Could you check a few things on this model? Use its own coordinates, in mm. Give positions to 0.01 mm unless a question says otherwise; leave off trailing zeros. Loops run counter-clockwise (first coordinate to the right, second up) from the corner with the lowest first, then second, coordinate; pieces in that order, holes last. Notation, with made-up numbers: M 36,57 L 45,57 A23 ccw 45,90 Z; hole C 64,85 d9. An arc over 180 degrees is marked long. Return JSON: item names as keys, results as strings. Group by question number.
1. If we section it at B-B (y = -64): Write out the boundary of the cut face in (x, z).
2. Please list where these lines run through material, in increasing order: line 1 (Z direction, x = 1.5, y = 6) (3 decimals); line 2 (Z direction, x = 1, y = 20); line 3 (Z direction, x = 1, y = -83.5).
3. If we section it at C-C (z = 23): Write out the boundary of the cut face in (x, y), plus the area to 3 significant figures.
4. If we section it at A-A (y = -19): Write out the boundary of the cut face in (x, z).
5. For pin 1 (1.3 mm diameter, centred on x = 3.5, z = 41, fed in from -Y); pin 2 (3 mm diameter, centred on x = 2, y = 4.5, fed in from -Z); pin 3 (0.7 mm diameter, centred on x = 2, z = 41, fed in from +Y), each with a flat end and sliding along its axis, tell me the tip position at first contact or that it passes through.
```python
from build123d import *

# Parameters (mm, degrees)
BOSS_EXTRUDE1_DEPTH = 6.35
CUT_EXTRUDE1_START  = -7.35
CUT_EXTRUDE1_DEPTH  = 8.35
LPATTERN1_COUNT     = 2
LPATTERN1_PITCH     = 19.05
CUT_EXTRUDE2_START  = -7.35
CUT_EXTRUDE2_DEPTH  = 8.35
CIRPATTERN2_COUNT   = 8
CIRPATTERN2_ANGLE   = 180
FILLET1_R           = 2.54


with BuildPart() as part:
    # Sketch1 → Boss-Extrude1 (new body)
    with BuildSketch(Plane(origin=(0, 0, 0), x_dir=(0, 0, -1), z_dir=(1, 0, 0))):
        with BuildLine():
            Line((-63.5, -98.425), (-63.5, 1.27))
            ThreePointArc((-63.5, 1.27), (-6.13650031, 61.522262538), (56.859225559, 7.185858903))
            Line((56.859225559, 7.185858903), (58.947868709, -14.009723349))
            ThreePointArc((58.947868709, -14.009723349), (54.036813814, -20.824301776), (46.661428403, -16.804273249))
            Line((46.661428403, -16.804273249), (35.802288852, 13.030967461))
            ThreePointArc((35.802288852, 13.030967461), (-6.615995569, 37.52117539), (-38.1, 0))
            Line((-38.1, 0), (-38.1, -98.425))
            ThreePointArc((-38.1, -98.425), (-50.8, -111.125), (-63.5, -98.425))
        make_face()
    extrude(amount=BOSS_EXTRUDE1_DEPTH)

    # Sketch4 → Cut-Extrude1 (cut)
    with BuildSketch(Plane(origin=(6.35, 0, 0), x_dir=(0, 0, -1), z_dir=(1, 0, 0)).offset(CUT_EXTRUDE1_START)):
        Polygon((44.489600492, -10.837225107), (47.473124563, -9.751311152), (45.301296653, -3.78426301), (42.317772582, -4.870176965), align=None)
    cut_extrude1 = extrude(amount=CUT_EXTRUDE1_DEPTH, mode=Mode.SUBTRACT)

    # LPattern1: Cut-Extrude1 ×2
    with Locations(*[Vector(0, 0.939692621, 0.342020143) * (i * LPATTERN1_PITCH) for i in range(1, LPATTERN1_COUNT)]):
        add(cut_extrude1, mode=Mode.SUBTRACT)

    # Sketch5 → Cut-Extrude2 (cut)
    with BuildSketch(Plane(origin=(6.35, 0, 0), x_dir=(0, 0, -1), z_dir=(1, 0, 0)).offset(CUT_EXTRUDE2_START)):
        Polygon((-38.1, 0), (-41.275, 0), (-41.275, 6.35), (-38.1, 6.35), (-35.06174314, 6.35), (-35.06174314, 0), align=None)
    cut_extrude2 = extrude(amount=CUT_EXTRUDE2_DEPTH, mode=Mode.SUBTRACT)

    # CirPattern2: Cut-Extrude2 ×8 about axis, 1 skipped
    cirpattern2_axis = Axis((0, 0, 0), (-1, 0, 0))
    add([cut_extrude2.rotate(cirpattern2_axis, i * CIRPATTERN2_ANGLE / (CIRPATTERN2_COUNT - 1)) for i in range(1, CIRPATTERN2_COUNT) if i not in (7,)], mode=Mode.SUBTRACT)

    # Fillet1
    fillet1_edges = [part.edges().sort_by_distance(p)[0] for p in [
        (3.175, 16.53097046, 34.326913867),
        (3.175, 22.020909, 31.091631781),
        (3.175, 29.787779482, 23.754961451),
        (3.175, 33.330306905, 18.458077951),
        (3.175, 37.144753454, 8.478047584),
        (3.175, 38.038228757, 2.168675409),
        (3.175, 37.144753454, -8.478047584),
        (3.175, 0, 38.1),
        (3.175, 35.212212896, -14.550259894),
        (3.175, 29.787779482, -23.754961451),
        (3.175, 25.411986421, -28.387337778),
        (3.175, 16.53097046, -34.326913867),
        (3.175, -10.837225107, -44.489600492),
        (3.175, -4.870176965, -42.317772582),
        (3.175, 7.063919319, -37.974116762),
        (3.175, 6.35, 37.567106623),
    ]]
    fillet(fillet1_edges, radius=FILLET1_R)


solid = part.part
```
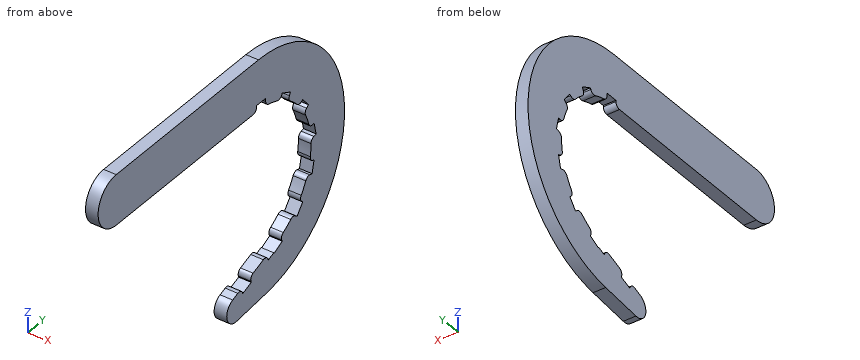
Answer:
{
 "1": {"outline": "M 0,38.1 L 6.35,38.1 L 6.35,63.5 L 0,63.5 Z"},
 "2": {"line 1": "z = -56.976 to -38.731, 41.275 to 63.314", "line 2": "z = -54.17 to -32.43, 36.18 to 60.52", "line 3": "z = 38.1 to 63.5"},
 "3": {"outline": "M 0,34.45 L 6.35,34.45 L 6.35,58.24 L 0,58.24 Z", "area": "151 mm²"},
 "4": {"outline": "M 0,-57.24 L 6.35,-57.24 L 6.35,-48.02 L 0,-48.02 Z; M 0,38.1 L 6.35,38.1 L 6.35,63.5 L 0,63.5 Z"},
 "5": {"pin 1": "stops at y = -107.23", "pin 2": "stops at z = -57.27", "pin 3": "stops at y = 48.54"}
}
